from build123d import *

# Parameters (mm, degrees)
SKETCH1_W           = 30
SKETCH1_H           = 27.727272728
BOSS_EXTRUDE1_DEPTH = 2
SKETCH2_W           = 10.248894408
SKETCH2_H           = 19.156033471
CUT_EXTRUDE1_DEPTH  = 2
FILLET1_R           = 0.5
FILLET2_R           = 0.5
FILLET3_R           = 0.5
FILLET4_R           = 0.5
FILLET5_R           = 0.5
SKETCH3_W           = 9.871005128
SKETCH3_H           = 10.546548519
BOSS_EXTRUDE2_DEPTH = 2


with BuildPart() as part:
    # Sketch1 → Boss-Extrude1 (new body)
    with BuildSketch(Plane.XY):
        Rectangle(SKETCH1_W, SKETCH1_H)
    extrude(amount=BOSS_EXTRUDE1_DEPTH)

    # Sketch2 → Cut-Extrude1 (cut)
    with BuildSketch(Plane.XY.offset(2)):
        with Locations((0, -4.294276099)):
            Rectangle(SKETCH2_W, SKETCH2_H)
    extrude(amount=-CUT_EXTRUDE1_DEPTH, mode=Mode.SUBTRACT)

    # Fillet1
    fillet1_edges = [part.edges().sort_by_distance(p)[0] for p in [
        (-15, 0, 2),
    ]]
    fillet(fillet1_edges, radius=FILLET1_R)

    # Fillet2
    fillet2_edges = [part.edges().sort_by_distance(p)[0] for p in [
        (15, 0, 2),
    ]]
    fillet(fillet2_edges, radius=FILLET2_R)

    # Fillet3
    fillet3_edges = [part.edges().sort_by_distance(p)[0] for p in [
        (-5.124447204, -4.289947863, 2),
    ]]
    fillet(fillet3_edges, radius=FILLET3_R)

    # Fillet4
    fillet4_edges = [part.edges().sort_by_distance(p)[0] for p in [
        (5.124447204, -4.289947863, 2),
    ]]
    fillet(fillet4_edges, radius=FILLET4_R)

    # Fillet5
    fillet5_edges = [part.edges().sort_by_distance(p)[0] for p in [
        (0, 5.283740637, 2),
    ]]
    fillet(fillet5_edges, radius=FILLET5_R)

    # Sketch3 → Boss-Extrude2 (add)
    with BuildSketch(Plane(origin=(0, -13.863636364, 0), x_dir=(-1, 0, 0), z_dir=(0, -1, 0))):
        with Locations((10.064497436, -5.273274259)):
            Rectangle(SKETCH3_W, SKETCH3_H)
    extrude(amount=BOSS_EXTRUDE2_DEPTH)


solid = part.part
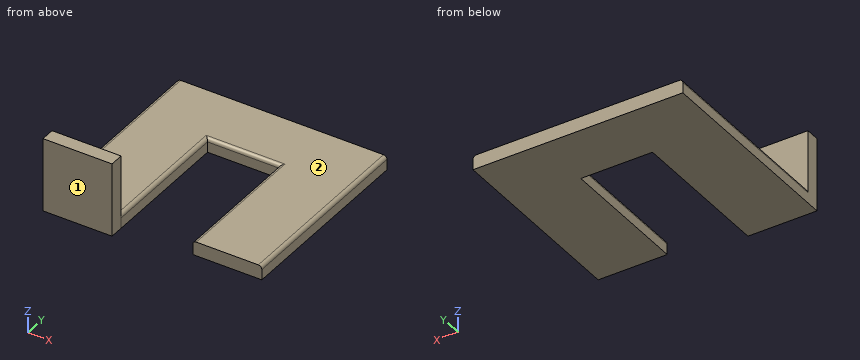
The listing builds one solid part. Answer for the finished solid, in the listing's coordinates (mm). Face numbers are marked on the shaded views. A direction names the side the tool comes from. Coordinates: 2 decimals unless noted, no trailing zeros. Write each loop counter-clockwise with the first axis right and the second up, starting at its lowest first coordinate (ties: lowest second). Pieces come first, ordered by that corner, then holes. Notation, with made-up numbers: M -39,65 L 7,65 A16 ccw 7,86 Z; hole C 64,43.25 d8. An arc over 180 degrees is marked long. Use one line per item in the form item = value.
Item 1: Find section D-D, the plane x = -9.5. Give the vertices of the cut face in (y, z), plus the area to 3 significant figures.
Model answer:
outline = M -15.86,0 L 13.86,0 L 13.86,2 L -13.86,2 L -13.86,10.55 L -15.86,10.55 Z
area = 76.5 mm2
Item 2: Find section A-A, the plane y = -13.25. Give the vertices of the cut face in (x, z).
Model answer:
outline = M -15,0 L -5.12,0 L -5.12,1.5 A0.5 ccw -5.62,2 L -14.5,2 A0.5 ccw -15,1.5 Z; M 5.12,0 L 15,0 L 15,1.5 A0.5 ccw 14.5,2 L 5.62,2 A0.5 ccw 5.12,1.5 Z
Item 3: Find section B-B, the plane x = -3. Give the vertices of the cut face in (y, z).
Model answer:
outline = M 5.28,0 L 13.86,0 L 13.86,2 L 5.78,2 A0.5 ccw 5.28,1.5 Z
Item 4: Given P1, Ø12, axis at x = -6, y = -4.5, coming from the +Z side; P2, Ø0.6, axis at y = -14.5, z = 7.5, coming from the +X side; P3, Ø0.6, axis at x = 10, z = 0.5, coming from the -Y side, each flat-ended and moving along its own axis, determine where each tip first touches the part or whether it passes through.
Model answer:
P1 = 2
P2 = -5.13
P3 = -13.86
Item 5: Find section C-C, the plane z = 9.5. Give the vertices of the cut face in (x, y), plus the area to 3 significant figures.
Model answer:
outline = M -15,-15.86 L -5.13,-15.86 L -5.13,-13.86 L -15,-13.86 Z
area = 19.7 mm2
Item 6: Find the intervals of material crossed by probe 1 along X at (y, z) = (4, 1.5); probe 2 along Z at (x, y) = (10.25, 0); probe 3 along Y at (x, z) = (-13, 9), in increasing order.
Model answer:
probe_1 = -15 to -5.12, 5.12 to 15
probe_2 = 0 to 2
probe_3 = -15.86 to -13.86
Item 7: For the marked faces 1 and 2, determine the directions among +Z, -Z, +X, -X, +Y, -Y from which every point of the face is accessible in a straight line to the end or side of a thin tool.
Model answer:
face_1 = +Z, -Z, +X, -X, -Y
face_2 = +Z, +X, -X, +Y
